```python
from build123d import *

# Parameters (mm, degrees)
F0_R      = 26.1
F0_R_2    = 23.1
F1_DEPTH  = 6
F3_DEPTH  = 2
F4_SIZE   = 1
F5_R      = 21.615
F5_R_2    = 18.615
F6_DEPTH  = 6
F8_DEPTH  = 2
F9_SIZE   = 1
F10_R     = 15.7
F10_R_2   = 12.7
F11_DEPTH = 6
F13_DEPTH = 2
F14_SIZE  = 1
F15_R     = 8
F15_R_2   = 5
F16_DEPTH = 6
F17_SIZE  = 1.5
F18_R     = 3


with BuildPart() as f1:
    # F0 (on Top) → F1 (new body)
    with BuildSketch(Plane.XY):
        with Locations((0, 234.9011148272)):
            Circle(F0_R)
        with Locations((0, 234.9011148272)):
            Circle(F0_R_2, mode=Mode.SUBTRACT)
    extrude(amount=F1_DEPTH)

    # F2 (on Top) → F3 (join)
    with BuildSketch(Plane.XY):
        with BuildLine():
            ThreePointArc((-19.8014794389, 240.2069052518), (-14.4956890143, 249.3968038415), (-5.3057904246, 254.7025942661))
            Line((-5.3057904246, 254.7025942661), (-5.9787199419, 257.2140014145))
            ThreePointArc((-5.9787199419, 257.2140014145), (-16.3341666454, 251.2352814726), (-22.3128865873, 240.8798347691))
            Line((-22.3128865873, 240.8798347691), (-19.8014794389, 240.2069052518))
        make_face()
        with BuildLine():
            ThreePointArc((5.3057904246, 254.7025942661), (14.4956890143, 249.3968038415), (19.8014794389, 240.2069052518))
            Line((19.8014794389, 240.2069052518), (22.3128865873, 240.8798347691))
            ThreePointArc((22.3128865873, 240.8798347691), (16.3341666454, 251.2352814726), (5.9787199419, 257.2140014145))
            Line((5.9787199419, 257.2140014145), (5.3057904246, 254.7025942661))
        make_face()
        with BuildLine():
            Line((22.3128865873, 228.9223948853), (19.8014794389, 229.5953244026))
            ThreePointArc((19.8014794389, 229.5953244026), (14.4956890143, 220.4054258129), (5.3057904246, 215.0996353883))
            Line((5.3057904246, 215.0996353883), (5.9787199419, 212.5882282399))
            ThreePointArc((5.9787199419, 212.5882282399), (16.3341666454, 218.5669481818), (22.3128865873, 228.9223948853))
        make_face()
        with BuildLine():
            Line((-5.9787199419, 212.5882282399), (-5.3057904246, 215.0996353883))
            ThreePointArc((-5.3057904246, 215.0996353883), (-14.4956890143, 220.4054258129), (-19.8014794389, 229.5953244026))
            Line((-19.8014794389, 229.5953244026), (-22.3128865873, 228.9223948853))
            ThreePointArc((-22.3128865873, 228.9223948853), (-16.3341666454, 218.5669481818), (-5.9787199419, 212.5882282399))
        make_face()
    extrude(amount=F3_DEPTH)

    # F4
    f4_edges = [f1.edges().sort_by_distance(p)[0] for p in [
        (-14.495689, 249.396804, 2),
        (14.495689, 249.396804, 2),
        (14.495689, 220.405426, 2),
        (-14.495689, 220.405426, 2),
    ]]
    chamfer(f4_edges, length=F4_SIZE)

    # F5 (on Top) → F6 (join)
    with BuildSketch(Plane.XY):
        with Locations((0, 189.1861148272)):
            Circle(F5_R)
        with Locations((0, 189.1861148272)):
            Circle(F5_R_2, mode=Mode.SUBTRACT)
    extrude(amount=F6_DEPTH)

    # F7 (on Top) → F8 (join)
    with BuildSketch(Plane.XY):
        with BuildLine():
            ThreePointArc((-15.469302108, 193.3311018345), (-11.3243151007, 200.5104299279), (-4.1449870073, 204.6554169352))
            Line((-4.1449870073, 204.6554169352), (-4.8179165246, 207.1668240836))
            ThreePointArc((-4.8179165246, 207.1668240836), (-13.1627927318, 202.348907559), (-17.9807092564, 194.0040313518))
            Line((-17.9807092564, 194.0040313518), (-15.469302108, 193.3311018345))
        make_face()
        with BuildLine():
            Line((4.8179165246, 207.1668240836), (4.1449870073, 204.6554169352))
            ThreePointArc((4.1449870073, 204.6554169352), (11.3243151007, 200.5104299279), (15.469302108, 193.3311018345))
            Line((15.469302108, 193.3311018345), (17.9807092564, 194.0040313518))
            ThreePointArc((17.9807092564, 194.0040313518), (13.1627927318, 202.348907559), (4.8179165246, 207.1668240836))
        make_face()
        with BuildLine():
            Line((17.9807092564, 184.3681983026), (15.469302108, 185.0411278199))
            ThreePointArc((15.469302108, 185.0411278199), (11.3243151007, 177.8617997265), (4.1449870073, 173.7168127192))
            Line((4.1449870073, 173.7168127192), (4.8179165246, 171.2054055708))
            ThreePointArc((4.8179165246, 171.2054055708), (13.1627927318, 176.0233220954), (17.9807092564, 184.3681983026))
        make_face()
        with BuildLine():
            Line((-4.8179165246, 171.2054055708), (-4.1449870073, 173.7168127192))
            ThreePointArc((-4.1449870073, 173.7168127192), (-11.3243151007, 177.8617997265), (-15.469302108, 185.0411278199))
            Line((-15.469302108, 185.0411278199), (-17.9807092564, 184.3681983026))
            ThreePointArc((-17.9807092564, 184.3681983026), (-13.1627927318, 176.0233220954), (-4.8179165246, 171.2054055708))
        make_face()
    extrude(amount=F8_DEPTH)

    # F9
    f9_edges = [f1.edges().sort_by_distance(p)[0] for p in [
        (-11.324315, 200.51043, 2),
        (11.324315, 200.51043, 2),
        (11.324315, 177.8618, 2),
        (-11.324315, 177.8618, 2),
    ]]
    chamfer(f9_edges, length=F9_SIZE)

    # F10 (on Top) → F11 (join)
    with BuildSketch(Plane.XY):
        with Locations((0, 154.8711148272)):
            Circle(F10_R)
        with Locations((0, 154.8711148272)):
            Circle(F10_R_2, mode=Mode.SUBTRACT)
    extrude(amount=F11_DEPTH)

    # F12 (on Top) → F13 (join)
    with BuildSketch(Plane.XY):
        with BuildLine():
            Line((-2.6140723555, 164.6269656727), (-3.2870018728, 167.1383728211))
            ThreePointArc((-3.2870018728, 167.1383728211), (-8.9802561211, 163.8513709483), (-12.2672579939, 158.1581167))
            Line((-12.2672579939, 158.1581167), (-9.7558508455, 157.4851871827))
            ThreePointArc((-9.7558508455, 157.4851871827), (-7.14177849, 162.0128933172), (-2.6140723555, 164.6269656727))
        make_face()
        with BuildLine():
            Line((3.2870018728, 167.1383728211), (2.6140723555, 164.6269656727))
            ThreePointArc((2.6140723555, 164.6269656727), (7.14177849, 162.0128933172), (9.7558508455, 157.4851871827))
            Line((9.7558508455, 157.4851871827), (12.2672579939, 158.1581167))
            ThreePointArc((12.2672579939, 158.1581167), (8.9802561211, 163.8513709483), (3.2870018728, 167.1383728211))
        make_face()
        with BuildLine():
            Line((12.2672579939, 151.5841129544), (9.7558508455, 152.2570424717))
            ThreePointArc((9.7558508455, 152.2570424717), (7.14177849, 147.7293363372), (2.6140723555, 145.1152639817))
            Line((2.6140723555, 145.1152639817), (3.2870018728, 142.6038568333))
            ThreePointArc((3.2870018728, 142.6038568333), (8.9802561211, 145.8908587061), (12.2672579939, 151.5841129544))
        make_face()
        with BuildLine():
            Line((-3.2870018728, 142.6038568333), (-2.6140723555, 145.1152639817))
            ThreePointArc((-2.6140723555, 145.1152639817), (-7.14177849, 147.7293363372), (-9.7558508455, 152.2570424717))
            Line((-9.7558508455, 152.2570424717), (-12.2672579939, 151.5841129544))
            ThreePointArc((-12.2672579939, 151.5841129544), (-8.9802561211, 145.8908587061), (-3.2870018728, 142.6038568333))
        make_face()
    extrude(amount=F13_DEPTH)

    # F14
    f14_edges = [f1.edges().sort_by_distance(p)[0] for p in [
        (-7.141778, 162.012893, 2),
        (7.141778, 162.012893, 2),
        (7.141778, 147.729336, 2),
        (-7.141778, 147.729336, 2),
    ]]
    chamfer(f14_edges, length=F14_SIZE)

    # F15 (on Top) → F16 (join)
    with BuildSketch(Plane.XY):
        with Locations((0, 132.1710638065)):
            Circle(F15_R)
        with Locations((0, 132.1710638065)):
            Circle(F15_R_2, mode=Mode.SUBTRACT)
    extrude(amount=F16_DEPTH)

    # F17
    f17_edges = [f1.edges().sort_by_distance(p)[0] for p in [
        (-5, 132.171064, 6),
    ]]
    chamfer(f17_edges, length=F17_SIZE)

    # F18
    f18_edges = [f1.edges().sort_by_distance(p)[0] for p in [
        (-6.801865, 209.703007, 3),
        (6.801865, 209.703007, 3),
        (7.219852, 168.812554, 3),
        (-7.219852, 168.812554, 3),
        (3.20387, 139.501495, 3),
        (-3.20387, 139.501495, 3),
    ]]
    fillet(f18_edges, radius=F18_R)


solid = f1.part
```
Geometry: final body of the model. Coordinates: model frame, mm. A direction names the side the tool comes from. Give positions to 0.01 mm unless a question says otherwise; leave off trailing zeros. Order: outer loops, then holes, each group sorted by start corner. A loop starts at its lowest first (then second) coordinate and runs counter-clockwise, first axis right, second up. Notation, with made-up numbers: (79, -32.75) -> (135, -32.75) arc R28 cw to (135, -9.75) -> close; hole circle Ø11 at (45, 37.5). An arc over 180 degrees is marked (long way). Write each question's results on one line, items separated by ' | '. Start each with the question number.
1) Section C-C (z = 3). Count the separate pieces of the cut face and the enclosed holes in it, then the cut area to 3 significant figures.
2) Line query: line 1 (Y direction, x = 0.5, z = 4); line 2 (X direction, y = 132, z = 4.5); line 3 (Y direction, x = 4, z = 5). Output: solid intervals per line, ascending. Write a range as from..to.
3) Section B-B (y = 233.5). Return loops of the section in (x, z).
4) Set-up query: faces 1 (the cylindrical face through (14.39, 249.5, 0.49)), 2 (the cylindrical face through (-21.614, 188.952, 2.958)), 3 (the conical face through (-14.501, 220.186, 1.16)). Return all of +Z, -Z, +X, -X, +Y, -Y with unobstructed straight access to the full face (end or side cutting, diameter ignored); none if empty.
5) First-contact query: pin 1 (3 mm diameter, centred on x = -5, z = 4, fed in from +Y); pin 2 (2 mm diameter, centred on x = 16, z = 3.5, fed in from +Y); pin 3 (1.5 mm diameter, centred on y = 175, z = 1.5, fed in from +X). Flat tips, straight axial feed; report the tip coordinate or a pass-through.
6) Section A-A (x = 0). Return loops of the section in (y, z), then the cut area to 3 significant figures.
Calculated:
1) separate pieces: 1 | enclosed holes: 4 | area: 1,210 mm2
2) line 1: 124.19..127.2, 137.15..142.18, 167.56..170.58, 207.79..211.81, 258..261 | line 2: -8..-5, 5..8 | line 3: 125.24..128.4, 135.95..142.82, 166.92..171.01, 207.37..212.15, 257.65..260.69
3) outline: (-26.06, 0) -> (-23.06, 0) -> (-23.06, 6) -> (-26.06, 6) -> close; (23.06, 0) -> (26.06, 0) -> (26.06, 6) -> (23.06, 6) -> close
4) face 1: +Z, -Z | face 2: +Z, -Z, -X | face 3: +Z
5) pin 1: y = 260.77 | pin 2: y = 256.26 | pin 3: x = 16.93
6) outline: (124.17, 0) -> (127.17, 0) -> (127.17, 4.5) -> (125.67, 6) -> (124.17, 6) -> close; (137.17, 0) -> (142.17, 0) -> (142.17, 6) -> (138.67, 6) -> (137.17, 4.5) -> close; (167.57, 0) -> (170.57, 0) -> (170.57, 6) -> (167.57, 6) -> close; (207.8, 0) -> (211.8, 0) -> (211.8, 6) -> (207.8, 6) -> close; (258, 0) -> (261, 0) -> (261, 6) -> (258, 6) -> close | area: 106 mm2
